Here's the drawing with two shaded views (mm, measured from the low corner). I have some questions. A direction names the side the tool comes from. Give positions to 0.01 mm unless a question says otherwise; leave off trailing zeros. Loops run counter-clockwise (first coordinate to the right, second up) from the corner with the lowest first, then second, coordinate; pieces in that order, holes last. Notation, with made-up numbers: M 0,-3.75 L 45,-3.75 A13 ccw 45,17.25 Z; hole C 77.5,-7 d11. An arc over 180 degrees is marked long. Answer in a Markdown table with one row per item. Add a question column.
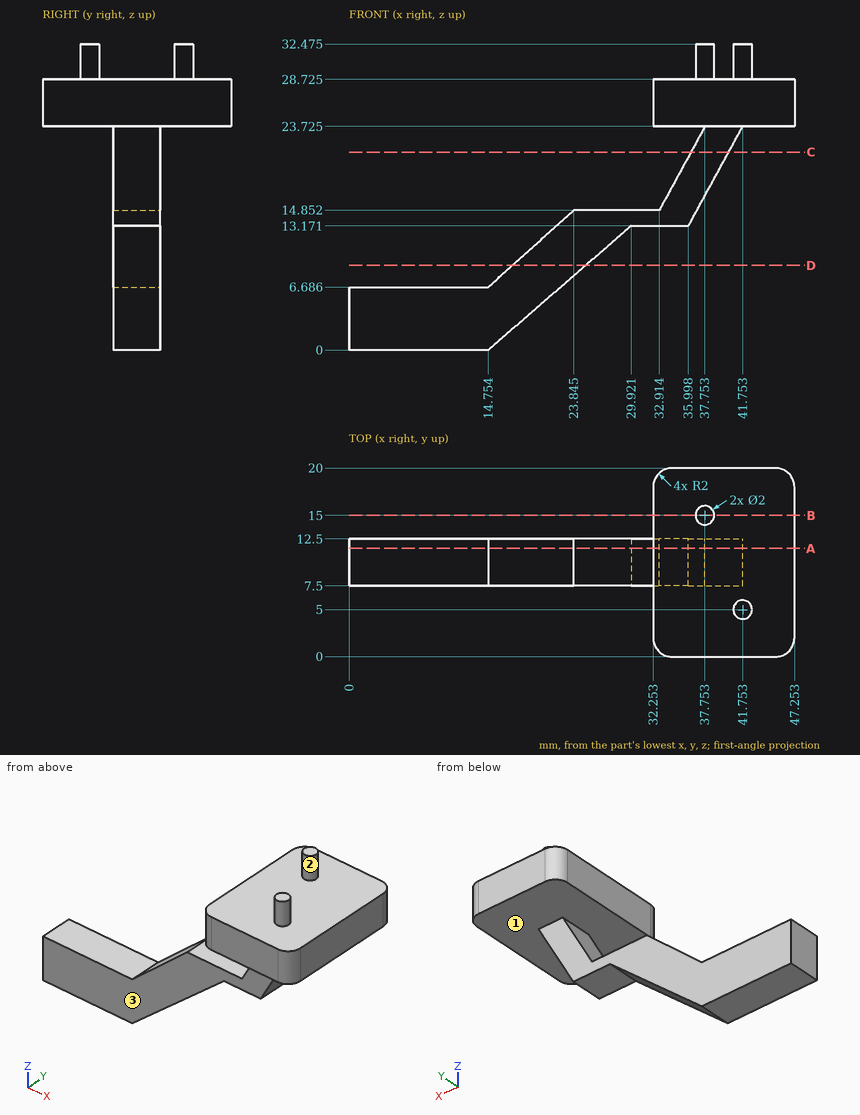
Item 1: For P1, Ø12, axis at y = 4, z = 26.5, coming from the -X side; P2, Ø6, axis at x = 5, y = 14.5, coming from the +Z side; P3, Ø2, axis at y = 14, z = 7, coming from the -X side; P4, Ø5.5, axis at x = 33, y = 10, coming from the -Z side, each with a flat end and sliding along its axis, tell me the tip position at first contact or that it passes through.
Item 2: Suppose I cut it at B-B (y = 15). List the corners of the cut face in (x, z) for me (1 decimal), then the cut area to 3 significant figures.
Item 3: I need wall thicknesses on L1, parallel to Z at x = 38, y = 13 (1 decimal); L2, parallel to Y at x = 24, z = 14; L3, parallel to X at y = 6.75, z = 27. Which ranges of each line are inside material? Lowest first, please.
Item 4: Suppose I cut it at C-C (z = 21). List the corners of the cut face in (x, y) for me.
Item 5: Suppose I cut it at A-A (y = 11.5). List the corners of the cut face in (x, z) for me (1 decimal).
Item 6: Suppose I cut it at D-D (z = 9). List the corners of the cut face in (x, y) for me.
Item 7: For the marked faces 1, 2 and 3, which set-ups out of +Z, -Z, +X, -X, +Y, -Y let a thin tool reach every point of the face, with its end or its side?
Values found:
| question | item | result |
|---|---|---|
| 1 | P1 | x = 32.25 |
| 1 | P2 | z = 6.69 |
| 1 | P3 | through |
| 1 | P4 | z = 13.17 |
| 2 | outline | M 32.3,23.7 L 47.3,23.7 L 47.3,28.7 L 38.8,28.7 L 38.8,32.5 L 36.8,32.5 L 36.8,28.7 L 32.3,28.7 Z |
| 2 | area | 82.5 mm² |
| 3 | L1 | 23.7 to 28.7 |
| 3 | L2 | 7.5 to 12.5 |
| 3 | L3 | 32.25 to 47.25 |
| 4 | outline | M 36.27,7.5 L 40.27,7.5 L 40.27,12.5 L 36.27,12.5 Z |
| 5 | outline | M 0,0 L 14.8,0 L 29.9,13.2 L 36,13.2 L 41.8,23.7 L 47.3,23.7 L 47.3,28.7 L 32.3,28.7 L 32.3,23.7 L 37.8,23.7 L 32.9,14.9 L 23.8,14.9 L 14.8,6.7 L 0,6.7 Z |
| 6 | outline | M 17.33,7.5 L 25.12,7.5 L 25.12,12.5 L 17.33,12.5 Z |
| 7 | face 1 | none |
| 7 | face 2 | +Z |
| 7 | face 3 | -Z, +X, -X, -Y |
